Autodesk Inventor part; units mm, degrees
ref_plane "YZ Plane" through (0, 0, 0) normal (1, 0, 0) x (0, 1, 0)
ref_plane "XZ Plane" through (0, 0, 0) normal (0, 1, 0) x (-1, 0, 0)
ref_plane "XY Plane" through (0, 0, 0) normal (0, 0, 1) x (1, 0, 0)
sketch "Sketch1" plane through (0, 0, 0) normal (0, 0, 1) x (1, 0, 0)
  circle A0 centre (0, 0) radius 2.5
  dimension "d0" = 5
extrude "Extrusion1" add sketch "Sketch1" along normal mid plane 20
chamfer "Chamfer1" distance 0.5 angle 45 2 edges at (-2.5, 0, 10) (-2.5, 0, -10)
sketch "Sketch2" plane through (0, 0, 0) normal (0, 0, 1) x (1, 0, 0)
  circle A0 centre (0, 0) radius 2
  circle A1 centre (0, 0) radius 4
  dimension "d6" = 8
extrude "Extrusion2" add sketch "Sketch2" along normal mid plane 10
properties part number "Lock pin"
Could you check a few things on this model? Use its own coordinates, in mm. A direction names the side the tool comes from. Give positions to 0.01 mm unless a question says otherwise; leave off trailing zeros. Loops run counter-clockwise (first coordinate to the right, second up) from the corner with the lowest first, then second, coordinate; pieces in that order, holes last. Notation, with made-up numbers: (77, 88) -> (97, 88) arc R14 ccw to (97, 95) -> close; hole circle Ø4 at (60, -8.5). An arc over 180 degrees is marked (long way). Return JSON: item names as keys, results as strings.
Item 1: If we section it at D-D on x = -3: List the corners of the cut face in (y, z) for me, plus the area to 3 significant figures.
Geometry results:
{"outline": "(-2.65, -5) -> (2.65, -5) -> (2.65, 5) -> (-2.65, 5) -> close", "area": "52.9 mm²"}
Item 2: If we section it at C-C on z = -8.25: List the corners of the cut face in (x, y) for me.
Geometry results:
{"outline": "circle Ø5 at (0, 0)"}
Item 3: I need wall thicknesses on L1, parallel to Z at x = 3.25, y = 1.75; L2, parallel to Y at x = -1, z = -0.5; L3, parallel to X at y = -3, z = 4.5. Which ranges of each line are inside material? Lowest first, please. Write a range as from..to.
Geometry results:
{"L1": "z = -5..5", "L2": "y = -3.87..3.87", "L3": "x = -2.65..2.65"}
Item 4: Which directions (+Z, -Z, +X, -X, +Y, -Y) give clear straight access to the entire face, cutting with the end or side of a thin tool? Please do faces 1 (the flat face through (0, 0, 10)), 2 (the cylindrical face through (-0.54, 2.44, 7.22)), 3 (the flat face through (2, 2, -5)).
Geometry results:
{"face 1": "+Z, +X, -X, +Y, -Y", "face 2": "+Z", "face 3": "-Z"}
Item 5: I'm going to push a flat-ended pin straight in: pin 1 (3 mm diameter, centred on x = 2.5, z = -1, fed in from -Y). Where does the tip first touch, or does it pass through?
Geometry results:
{"pin 1": "stops at y = -3.87"}
Item 6: If we section it at A-A on y = 0: List the corners of the cut face in (x, z) for me, plus the area to 4 significant figures.
Geometry results:
{"outline": "(-4, -5) -> (-2.5, -5) -> (-2.5, -9.5) -> (-2, -10) -> (2, -10) -> (2.5, -9.5) -> (2.5, -5) -> (4, -5) -> (4, 5) -> (2.5, 5) -> (2.5, 9.5) -> (2, 10) -> (-2, 10) -> (-2.5, 9.5) -> (-2.5, 5) -> (-4, 5) -> close", "area": "129.5 mm²"}
